The figure shows three views and two pictorial views of one solid part (mm, origin at its lowest corner). Answer the questions. Coordinates: 2 decimals unless noted, no trailing zeros. Write each loop counter-clockwise with the first axis right and the second up, starting at its lowest first coordinate (ties: lowest second). Pieces come first, ordered by that corner, then holes.
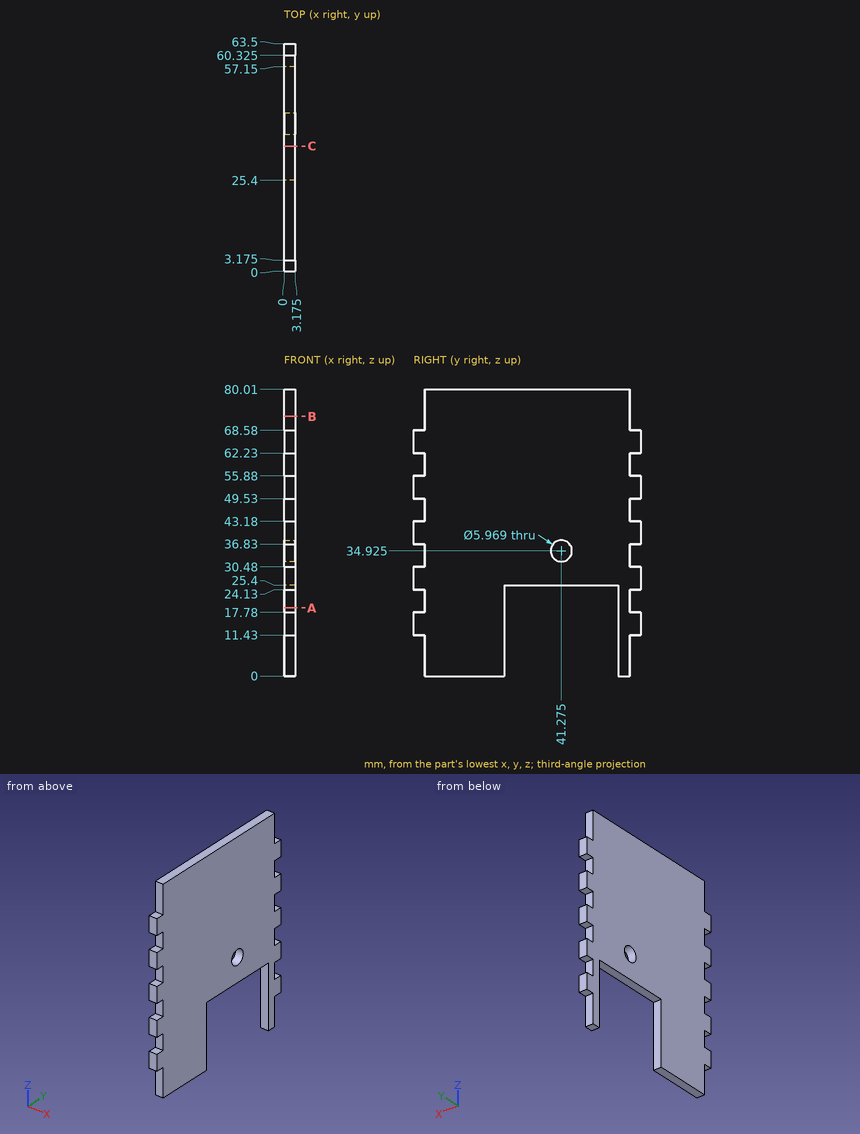
1. Find the intervals of material crossed by L1, parallel to Z at x = 0.5, y = 60.5; L2, parallel to Y at x = 0.35, z = 19 (3 decimals); L3, parallel to Y at x = 2.1, z = 12, in increasing order.
Results found:
L1: z = 11.43 to 17.78, 24.13 to 30.48, 36.83 to 43.18, 49.53 to 55.88, 62.23 to 68.58
L2: y = 3.175 to 25.4, 57.15 to 60.325
L3: y = 0 to 25.4, 57.15 to 63.5
2. Section A-A on z = 19 is taken. Give the vertices of the cut face in (x, y) (3 decimals).
Results found:
outline: (0, 3.175) - (3.175, 3.175) - (3.175, 25.4) - (0, 25.4) - close; (0, 57.15) - (3.175, 57.15) - (3.175, 60.325) - (0, 60.325) - close
3. Section C-C on y = 35 is taken. Give the vertices of the cut face in (x, z) (3 decimals).
Results found:
outline: (0, 25.4) - (3.175, 25.4) - (3.175, 80.01) - (0, 80.01) - close
4. Section B-B on z = 72.5 is taken. Give the vertices of the cut face in (x, y) (3 decimals), then the cut area to 3 significant figures.
Results found:
outline: (0, 3.175) - (3.175, 3.175) - (3.175, 60.325) - (0, 60.325) - close
area: 181 mm2
5. Flat-ended cylindrical pins translate along their axes: P1, Ø8, axis at y = 41.275, z = 34.925, coming from the +X side (3 decimals); P2, Ø1.6, axis at x = 2, z = 33, coming from the +Y side (3 decimals); P3, Ø1.6, axis at x = 1.5, y = 61.5, coming from the +Z side; P4, Ø1.6, axis at x = 1, y = 2, coming from the -Z side. Find the tip coordinate at first contact, or state that the pin passes through.
Results found:
P1: stops at x = 3.175
P2: stops at y = 60.325
P3: stops at z = 68.58
P4: stops at z = 11.43
